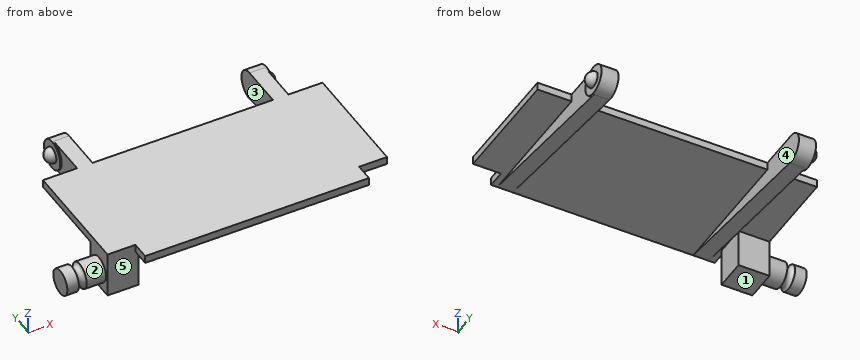
from build123d import *

# Parameters (mm, degrees)
PAD038_DEPTH             = 1
PAD039_DEPTH             = 2.2
POCKET022_DEPTH          = 0.2
PAD040_DEPTH             = 2.2
POCKET023_DEPTH          = 0.2
SKETCH063_W              = 4
SKETCH063_H              = 4
PAD041_DEPTH             = 5
SKETCH064_R              = 1.65
PAD042_DEPTH             = 5
SKETCH065_R              = 0.5
PAD084_DEPTH             = 2
PAD085_DEPTH             = 2
CLONE003_PLACEMENT_ANGLE = 180


with BuildPart() as part:
    # Sketch058 (on DatumPlane) → Pad038 (new body)
    with BuildSketch(Plane(origin=(0, 0, -0.6), x_dir=(1, 0, 0), z_dir=(0, 0, -1))):
        Polygon((45.85, -61.65), (45.85, -76.8), (49.45, -76.8), (49.45, -79.1), (78.35, -79.1), (78.35, -76.8), (81.95, -76.8), (81.95, -61.65), (77.55, -61.65), (77.55, -58.65), (77.75, -58.65), (77.75, -56.15), (75.55, -56.15), (75.55, -61.65), (52.25, -61.65), (52.25, -56.15), (50.05, -56.15), (50.05, -58.65), (50.25, -58.65), (50.25, -61.65), align=None)
    extrude(amount=PAD038_DEPTH)

    # Sketch059 (on Face17 of Pad038) → Pad039 (join)
    with BuildSketch(Plane(origin=(50.05, 0, -0.6), x_dir=(0, 1, 0), z_dir=(-1, 0, 0))):
        with BuildLine():
            ThreePointArc((57.82332, 1), (55.175321, 3.530951), (56.15, 0))
            Line((56.15, 1), (56.15, 0))
            Line((57.82332, 1), (56.15, 1))
        make_face()
    extrude(amount=-PAD039_DEPTH)

    # Sketch060 (on Face22 of Pad039) → Pocket022 (cut)
    with BuildSketch(Plane(origin=(50.05, 0, -0.6), x_dir=(0, 1, 0), z_dir=(-1, 0, 0))):
        with BuildLine():
            ThreePointArc((56.15, 0), (57.124679, 0.269049), (57.82332, 1))
            Line((57.82332, 1), (58.65, 1))
            Line((58.65, 1), (58.65, 0))
            Line((58.65, 0), (56.15, 0))
        make_face()
    extrude(amount=-POCKET022_DEPTH, mode=Mode.SUBTRACT)

    # Sketch061 (on Face14 of Pocket022) → Pad040 (join)
    with BuildSketch(Plane(origin=(77.75, 0, -0.6), x_dir=(0, -1, 0), z_dir=(1, 0, 0))):
        with BuildLine():
            ThreePointArc((-56.15, 0), (-55.175321, 3.530951), (-57.82332, 1))
            Line((-57.82332, 1), (-56.15, 1))
            Line((-56.15, 1), (-56.15, 0))
        make_face()
    extrude(amount=-PAD040_DEPTH)

    # Sketch062 (on Face20 of Pad040) → Pocket023 (cut)
    with BuildSketch(Plane(origin=(77.75, 0, -0.6), x_dir=(0, -1, 0), z_dir=(1, 0, 0))):
        with BuildLine():
            ThreePointArc((-57.82332, 1), (-57.124679, 0.269049), (-56.15, 0))
            Line((-58.65, 0), (-56.15, 0))
            Line((-58.65, 1), (-58.65, 0))
            Line((-57.82332, 1), (-58.65, 1))
        make_face()
    extrude(amount=-POCKET023_DEPTH, mode=Mode.SUBTRACT)

    # Sphere004 → Sphere004 (revolve)
    with BuildSketch(Plane(origin=(50.05, 56.15, -2.5), x_dir=(0, 1, 0), z_dir=(0, 0, -1))):
        with BuildLine():
            ThreePointArc((0, -1), (1, 0), (0, 1))
            Line((0, 1), (0, -1))
        make_face()
    revolve(axis=Axis((50.05, 56.15, -2.5), (1, 0, 0)))

    # Sphere005 → Sphere005 (revolve)
    with BuildSketch(Plane(origin=(77.75, 56.15, -2.5), x_dir=(0, 1, 0), z_dir=(0, 0, -1))):
        with BuildLine():
            ThreePointArc((0, -1), (1, 0), (0, 1))
            Line((0, 1), (0, -1))
        make_face()
    revolve(axis=Axis((77.75, 56.15, -2.5), (1, 0, 0)))

    # Sketch063 (on Face5 of Sphere005) → Pad041 (join)
    with BuildSketch(Plane(origin=(77.75, 56.15, -1.6), x_dir=(0, 1, 0), z_dir=(0, 0, -1))):
        with Locations((18.65, 2.2)):
            Rectangle(SKETCH063_W, SKETCH063_H)
    extrude(amount=PAD041_DEPTH)

    # Sketch064 (on Face25 of Pad041) → Pad042 (join)
    with BuildSketch(Plane(origin=(81.95, 56.15, -2.5), x_dir=(0, 1, 0), z_dir=(1, 0, 0))):
        with Locations((18.65, -1.599996)):
            Circle(SKETCH064_R)
    extrude(amount=PAD042_DEPTH)

    # Sketch065 (on DatumPlane) → Groove002 (revolve, cut)
    with BuildSketch(Plane(origin=(84.45, 74.8, -4.1), x_dir=(0, 1, 0), z_dir=(0, 0, -1))):
        with Locations((1.680544, 0.5)):
            Circle(SKETCH065_R)
    revolve(axis=Axis((84.45, 74.8, -4.1), (1, 0, 0)), mode=Mode.SUBTRACT)

    # Sketch107 (on Face17 of Groove002) → Pad084 (join)
    with BuildSketch(Plane(origin=(52.25, 56.15, -2.5), x_dir=(0, 1, 0), z_dir=(1, 0, 0))):
        Polygon((22.95, 0.900005), (0.231255, -1.885874), (1.67332, 0.9), align=None)
    extrude(amount=-PAD084_DEPTH)

    # Sketch108 (on Face14 of Pad084) → Pad085 (join)
    with BuildSketch(Plane(origin=(75.55, 56.15, -2.5), x_dir=(0, 1, 0), z_dir=(-1, 0, 0))):
        Polygon((1.67332, -0.9), (22.95, -0.900005), (0.231255, 1.885874), align=None)
    extrude(amount=-PAD085_DEPTH)


with BuildPart() as part_1:
    # Clone003 placement: moved
    add(part.part.moved(Location((91.8, 159.4, 0))).rotate(Axis((91.8, 159.4, 0), (0, 0, -1)), CLONE003_PLACEMENT_ANGLE))


with BuildPart() as part_2:
    # Body021 placement: moved
    add(part_1.part.moved(Location((36, 0, 0))))


solid = part_2.part
Verification items for the finished model (mm, model axes). Face numbers are marked on the shaded views. A direction names the side the tool comes from. Round coordinates to 2 decimals unless told otherwise and drop trailing zeros. Write each loop counter-clockwise with the first axis right and the second up, starting at its lowest first coordinate (ties: lowest second). Pieces come first, ordered by that corner, then holes.
(1) Section check B-B (x = 75). Enter the section's corners in (y, z), plus the area to 4 significant figures.
Returned:
outline: (80.3, -1.6) - (97.75, -1.6) - (97.75, -0.6) - (80.3, -0.6) - close
area: 17.45 mm2
(2) Section check A-A (y = 97.25). Enter the section's corners in (x, z), plus the area to 3 significant figures.
Returned:
outline: (45.85, -1.6) - (50.25, -1.6) - (50.25, -3.68) - (52.25, -3.68) - (52.25, -1.6) - (75.55, -1.6) - (75.55, -3.68) - (77.55, -3.68) - (77.55, -1.6) - (81.95, -1.6) - (81.95, -0.6) - (45.85, -0.6) - close
area: 44.4 mm2
(3) Section check C-C (y = 89.75). Enter the section's corners in (x, z).
Returned:
outline: (45.85, -1.6) - (50.25, -1.6) - (50.25, -2.76) - (52.25, -2.76) - (52.25, -1.6) - (75.55, -1.6) - (75.55, -2.76) - (77.55, -2.76) - (77.55, -1.6) - (81.95, -1.6) - (81.95, -0.6) - (45.85, -0.6) - close
(4) Depth check by flat-ended pin: pin 1 Ø2 at (y, z) = (100, -2.5) entering from -X; pin 2 Ø1.5 at (y, z) = (84.5, -5.5) entering from +X; pin 3 Ø2 at (x, z) = (48, -3.5) entering from -Y. Enter the tip coordinate at first touch or a pass-through.
Returned:
pin 1: stops at x = 50.25
pin 2: stops at x = 49.85
pin 3: stops at y = 82.6
(5) Material ranges on line 1 (X direction, y = 99.5, z = -0.75); line 2 (Z direction, x = 79.5, y = 91.5), recorded low to high.
Returned:
line 1: x = 50.25 to 52.25, 75.55 to 77.55
line 2: z = -1.6 to -0.6
(6) Mould release check, pull along X, two halves, no side actions. Record for the marked faces 3, 4 and 5: pulls with the +X half, pulls with the -X half, needs draft (parallel to the pull), parting line crosses it, or undercut.
Returned:
face 3: undercut
face 4: undercut
face 5: needs draft
(7) Section check D-D (y = 84.6). Enter the section's corners in (x, z).
Returned:
outline: (40.85, -5.75) - (42.35, -5.75) arc R0.5 cw to (43.35, -5.75) - (45.85, -5.75) - (45.85, -6.6) - (49.85, -6.6) - (49.85, -1.6) - (50.25, -1.6) - (50.25, -2.13) - (52.25, -2.13) - (52.25, -1.6) - (75.55, -1.6) - (75.55, -2.13) - (77.55, -2.13) - (77.55, -1.6) - (81.95, -1.6) - (81.95, -0.6) - (45.85, -0.6) - (45.85, -2.45) - (43.35, -2.45) arc R0.5 cw to (42.35, -2.45) - (40.85, -2.45) - close
(8) Access from +Z, -Z, +X, -X, +Y, -Y to the whole of each face (thin tool, end or side, straight path). Record for the marked faces 1 and 2.
Returned:
face 1: -Z, +X, -X, +Y, -Y
face 2: -X
